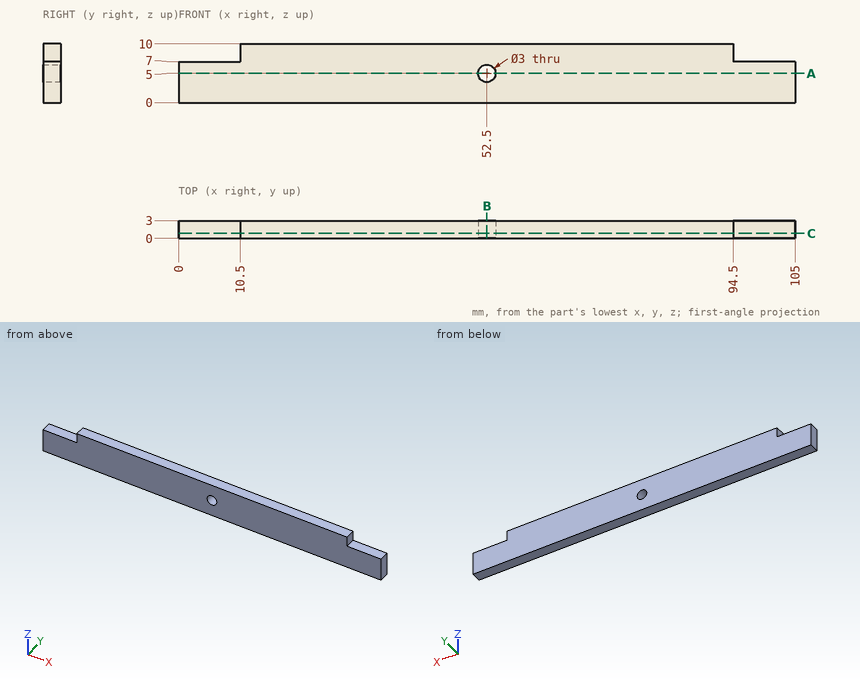
Verification items for this drawing (mm, ordinates from the low corner). Coordinates: 2 decimals unless noted, no trailing zeros. Order: outer loops, then holes, each group sorted by start corner. A loop starts at its lowest first (then second) coordinate and runs counter-clockwise, first axis right, second up. Notation, with made-up numbers: (13.5, 20.25) - (54.5, 20.25) arc R18 ccw to (54.5, 37.25) - close; hole circle Ø7 at (66.5, 14). An arc over 180 degrees is marked (long way). Use one line per item in the form item = value.
1. Scan lines: line 1 (X direction, y = 1.15, z = 5); line 2 (X direction, y = 0.4, z = 9); line 3 (X direction, y = 1.05, z = 4.5). Record each from-to range of solid material in increasing order.
Here are the results:
line_1 = 0 to 51, 54 to 105
line_2 = 10.5 to 94.5
line_3 = 0 to 51.09, 53.91 to 105
2. Section check A-A (z = 5). Record the boundary of the cut face in (x, y), then the cut area to 3 significant figures.
Here are the results:
outline = (0, 0) - (51, 0) - (51, 3) - (0, 3) - close; (54, 0) - (105, 0) - (105, 3) - (54, 3) - close
area = 306 mm²
3. Gauge pin test, flat ends, axial feed: pin 1 (1.5 mm diameter, centred on x = 98.5, y = 1.5, fed in from +Z); pin 2 (0.9 mm diameter, centred on y = 1, z = 8, fed in from +X); pin 3 (1.5 mm diameter, centred on y = 1.5, z = 8, fed in from -X); pin 4 (1 mm diameter, centred on x = 12.5, z = 5.5, fed in from -Y). Record the tip position at first contact, or that the pin passes through.
Here are the results:
pin_1 = 7
pin_2 = 94.5
pin_3 = 10.5
pin_4 = 0
4. Section check C-C (y = 0.85). Record the boundary of the cut face in (x, z).
Here are the results:
outline = (0, 0) - (105, 0) - (105, 7) - (94.5, 7) - (94.5, 10) - (10.5, 10) - (10.5, 7) - (0, 7) - close; hole circle Ø3 at (52.5, 5)
5. Section check B-B (x = 52.5). Record the boundary of the cut face in (y, z), then the cut area to 3 significant figures.
Here are the results:
outline = (0, 0) - (3, 0) - (3, 3.5) - (0, 3.5) - close; (0, 6.5) - (3, 6.5) - (3, 10) - (0, 10) - close
area = 21.0 mm²
